Input: part model. Units: mm. Frame: model coordinates. Face numbers are marked on the shaded views. A direction names the side the tool comes from. Round coordinates to 2 decimals unless told otherwise and drop trailing zeros. Write each loop counter-clockwise with the first axis right and the second up, starting at its lowest first coordinate (ties: lowest second). Pieces come first, ordered by that corner, then holes. Notation, with made-up numbers: (-33, 57) -> (11, 57) arc R7 ccw to (11, 61) -> close; hole circle Ø3 at (-35, -35). An arc over 180 degrees is marked (long way). Write item = value, one per line.
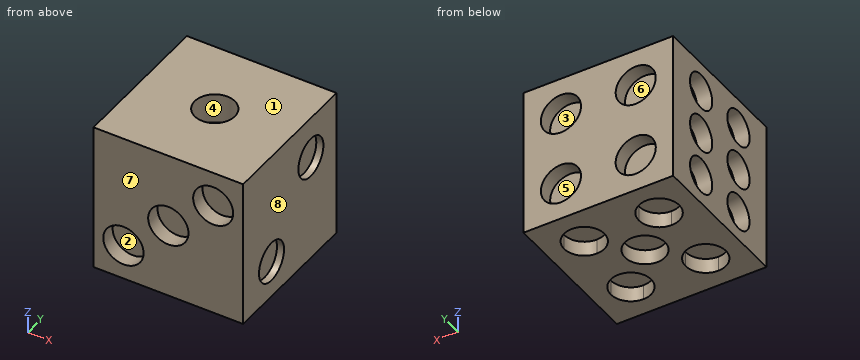
```python
from build123d import *

# Parameters (mm, degrees)
F0_R      = 3.405104
F1_DEPTH  = 25.4
F3_DEPTH  = 20.32
F4_R      = 3.422318
F4_R_2    = 3.418745
F4_R_3    = 3.399739
F5_DEPTH  = 2.54
F6_R      = 3.408954
F6_R_2    = 3.409845
F6_R_3    = 3.399812
F6_R_4    = 3.407384
F7_DEPTH  = 2.54
F9_DEPTH  = 2.54
F10_R     = 3.020938
F10_R_2   = 3.01106
F10_R_3   = 3.009838
F10_R_4   = 3.023548
F10_R_5   = 3.010431
F10_R_6   = 2.996939
F11_DEPTH = 2.54
F2_R      = 3.407459
F2_R_2    = 3.398087
F12_DEPTH = 2.54


with BuildPart() as f1:
    # F0 (on Top) → F1 (new body)
    with BuildSketch(Plane.XY):
        Polygon((-5.147523, 8.376352), (-22.927523, 8.376352), (-26.737523, 8.376352), (-26.737523, 4.566352), (-26.737523, -13.213648), (-26.737523, -17.023648), (-22.927523, -17.023648), (-5.147523, -17.023648), (-1.337523, -17.023648), (-1.337523, -13.213648), (-1.337523, 4.566352), (-1.337523, 8.376352), align=None)
        with Locations((-14.236085, -4.059524)):
            Circle(F0_R, mode=Mode.SUBTRACT)
    extrude(amount=F1_DEPTH)

    # F0 (on Top) → F3 (join)
    with BuildSketch(Plane.XY):
        with Locations((-14.236085, -4.059524)):
            Circle(F0_R)
    extrude(amount=F3_DEPTH)

    # F4 (on face) → F5 (cut)
    with BuildSketch(Plane.XZ.offset(17.023648)):
        with Locations((-21.657523, 5.979792)):
            Circle(F4_R)
        with Locations((-14.037523, 12.7)):
            Circle(F4_R_2)
        with Locations((-6.417523, 19.420208)):
            Circle(F4_R_3)
    extrude(amount=-F5_DEPTH, mode=Mode.SUBTRACT)

    # F6 (on face) → F7 (cut)
    with BuildSketch(Plane(origin=(0, 8.376352, 0), x_dir=(-1, 0, 0), z_dir=(0, 1, 0))):
        with Locations((7.687523, 19.05)):
            Circle(F6_R)
        with Locations((20.387523, 6.35)):
            Circle(F6_R_2)
        with Locations((20.387523, 19.05)):
            Circle(F6_R_3)
        with Locations((7.687523, 6.35)):
            Circle(F6_R_4)
    extrude(amount=-F7_DEPTH, mode=Mode.SUBTRACT)

    # F8 (on face) → F9 (cut)
    with BuildSketch(Plane(origin=(0, 0, 0), x_dir=(1, 0, 0), z_dir=(0, 0, -1))):
        with BuildLine():
            Line((-14.037523, 4.323648), (-10.639824, 4.323648))
            ThreePointArc((-10.639824, 4.323648), (-14.037523, 7.721346), (-17.435221, 4.323648))
            Line((-17.435221, 4.323648), (-14.037523, 4.323648))
        make_face()
        with BuildLine():
            ThreePointArc((-16.966481, -2.026352), (-17.968481, 0.392689), (-20.387523, 1.394689))
            Line((-20.387523, 1.394689), (-20.387523, -5.447394))
            ThreePointArc((-20.387523, -5.447394), (-17.968481, -4.445394), (-16.966481, -2.026352))
        make_face()
        with BuildLine():
            Line((-20.387523, -5.447394), (-20.387523, 1.394689))
            ThreePointArc((-20.387523, 1.394689), (-23.808564, -2.026352), (-20.387523, -5.447394))
        make_face()
        with BuildLine():
            ThreePointArc((-20.387523, 14.08974), (-23.803615, 10.673648), (-20.387523, 7.257555))
            Line((-20.387523, 7.257555), (-20.387523, 14.08974))
        make_face()
        with BuildLine():
            Line((-20.387523, 14.08974), (-20.387523, 7.257555))
            ThreePointArc((-20.387523, 7.257555), (-17.97198, 8.258105), (-16.97143, 10.673648))
            ThreePointArc((-16.97143, 10.673648), (-17.97198, 13.08919), (-20.387523, 14.08974))
        make_face()
        with BuildLine():
            ThreePointArc((-17.435221, 4.323648), (-14.037523, 0.925949), (-10.639824, 4.323648))
            Line((-10.639824, 4.323648), (-14.037523, 4.323648))
            Line((-14.037523, 4.323648), (-17.435221, 4.323648))
        make_face()
        with BuildLine():
            ThreePointArc((-7.687523, 14.080634), (-11.094509, 10.673648), (-7.687523, 7.266661))
            Line((-7.687523, 7.266661), (-7.687523, 14.080634))
        make_face()
        with BuildLine():
            Line((-7.687523, 14.080634), (-7.687523, 7.266661))
            ThreePointArc((-7.687523, 7.266661), (-5.278419, 8.264544), (-4.280536, 10.673648))
            ThreePointArc((-4.280536, 10.673648), (-5.278419, 13.082751), (-7.687523, 14.080634))
        make_face()
        with BuildLine():
            ThreePointArc((-4.270767, -2.026352), (-5.271512, 0.389659), (-7.687523, 1.390403))
            Line((-7.687523, 1.390403), (-7.687523, -5.443108))
            ThreePointArc((-7.687523, -5.443108), (-5.271512, -4.442363), (-4.270767, -2.026352))
        make_face()
        with BuildLine():
            Line((-7.687523, -5.443108), (-7.687523, 1.390403))
            ThreePointArc((-7.687523, 1.390403), (-11.104278, -2.026352), (-7.687523, -5.443108))
        make_face()
    extrude(amount=-F9_DEPTH, mode=Mode.SUBTRACT)

    # F10 (on face) → F11 (cut)
    with BuildSketch(Plane(origin=(-26.737523, 0, 0), x_dir=(0, -1, 0), z_dir=(-1, 0, 0))):
        with Locations((9.403648, 20.32)):
            Circle(F10_R)
        with Locations((9.403648, 12.7)):
            Circle(F10_R_2)
        with Locations((-0.756352, 12.699992)):
            Circle(F10_R_3)
        with Locations((-0.756352, 20.32)):
            Circle(F10_R_4)
        with Locations((-0.756352, 5.08)):
            Circle(F10_R_5)
        with Locations((9.403648, 5.08)):
            Circle(F10_R_6)
    extrude(amount=-F11_DEPTH, mode=Mode.SUBTRACT)

    # F2 (on Right) → F12 (cut)
    with BuildSketch(Plane.YZ):
        with Locations((-9.293744, 6.306227)):
            Circle(F2_R)
        with Locations((1.408402, 18.246217)):
            Circle(F2_R_2)
    extrude(amount=-F12_DEPTH, mode=Mode.SUBTRACT)


solid = f1.part
```
1) Line query: L1, parallel to X at y = -13.5, z = 2.5; L2, parallel to Y at x = -25.5, z = 3.5; L3, parallel to Z at x = -24.75, y = 2.5. Output: solid intervals per line, ascending. Write a range as from..to.
Solutions:
L1 = -26.74..-22.31, -18.47..-9.59, -5.79..-1.34
L2 = -17.02..-11.95, -6.86..-1.81, 3.32..8.38
L3 = 0..2.63, 7.53..10.25, 15.15..17.85, 22.79..25.4
2) First-contact query: P1, Ø3, axis at y = 0.5, z = 13, coming from the -X side; P2, Ø5.5, axis at x = -20, z = 19, coming from the +Y side; P3, Ø2, axis at x = -20, z = 7, coming from the -Y side. Flat tips, straight axial feed; report the tip coordinate or a pass-through.
Solutions:
P1 = -24.2
P2 = 5.84
P3 = -14.48
3) Draft query along X for the marked faces 5, 6, 7 and 8. Return one class per face: +X half, -X half, draft (parallel to the pull), parting line (faces both ways), or undercut.
Solutions:
face_5 = undercut
face_6 = undercut
face_7 = draft
face_8 = +X half
4) Access query for the marked faces 1, 2, 3 and 4. Directions: +Z, -Z, +X, -X, +Y, -Y. A direction counts if a zero-diameter tool reaches every point of the face in a straight line with its end or side. Return the directions, or none.
Solutions:
face_1 = +Z, +X, -X, +Y, -Y
face_2 = -Y
face_3 = +Y
face_4 = +Z
5) Cut plane A-A (x = -19.25). Return the cut outline in (y, z).
Solutions:
outline = (-17.02, 0) -> (-13.89, 0) -> (-13.89, 2.54) -> (-7.45, 2.54) -> (-7.45, 0) -> (-1.2, 0) -> (-1.2, 2.54) -> (5.25, 2.54) -> (5.25, 0) -> (8.38, 0) -> (8.38, 3.14) -> (5.84, 3.14) -> (5.84, 9.56) -> (8.38, 9.56) -> (8.38, 15.85) -> (5.84, 15.85) -> (5.84, 22.25) -> (8.38, 22.25) -> (8.38, 25.4) -> (-17.02, 25.4) -> (-17.02, 8.41) -> (-14.48, 8.41) -> (-14.48, 3.55) -> (-17.02, 3.55) -> close
6) Cut plane C-C (z = 8.5). Return the cut outline in (x, y), and give its area (3 significant figures).
Solutions:
outline = (-26.74, -17.02) -> (-23.97, -17.02) -> (-23.97, -14.48) -> (-19.34, -14.48) -> (-19.34, -17.02) -> (-1.34, -17.02) -> (-1.34, -11.9) -> (-2.54, -11.9) -> (-2.54, -6.69) -> (-1.34, -6.69) -> (-1.34, 8.38) -> (-5.04, 8.38) -> (-5.04, 5.84) -> (-10.33, 5.84) -> (-10.33, 8.38) -> (-17.74, 8.38) -> (-17.74, 5.84) -> (-23.03, 5.84) -> (-23.03, 8.38) -> (-26.74, 8.38) -> close
area = 600 mm^2
7) Cut plane D-D (x = -8.5). Return the cut outline in (y, z), and give its area (3 significant figures).
Solutions:
outline = (-17.02, 0) -> (-13.98, 0) -> (-13.98, 2.54) -> (-7.36, 2.54) -> (-7.36, 0) -> (-1.29, 0) -> (-1.29, 2.54) -> (5.35, 2.54) -> (5.35, 0) -> (8.38, 0) -> (8.38, 3.04) -> (5.84, 3.04) -> (5.84, 9.66) -> (8.38, 9.66) -> (8.38, 15.74) -> (5.84, 15.74) -> (5.84, 22.36) -> (8.38, 22.36) -> (8.38, 25.4) -> (-17.02, 25.4) -> (-17.02, 22.11) -> (-14.48, 22.11) -> (-14.48, 16.73) -> (-17.02, 16.73) -> close
area = 564 mm^2
8) Cut plane B-B (z = 14.25). Return the cut outline in (x, y), and give its area (3 significant figures).
Solutions:
outline = (-26.74, -17.02) -> (-17.08, -17.02) -> (-17.08, -14.48) -> (-10.99, -14.48) -> (-10.99, -17.02) -> (-1.34, -17.02) -> (-1.34, 8.38) -> (-26.74, 8.38) -> (-26.74, 3.34) -> (-24.2, 3.34) -> (-24.2, -1.82) -> (-26.74, -1.82) -> (-26.74, -6.82) -> (-24.2, -6.82) -> (-24.2, -11.99) -> (-26.74, -11.99) -> close
area = 603 mm^2
